Here's how the part is built. I have some questions about the finished solid (model axes, mm). Round coordinates to 2 decimals unless told otherwise and drop trailing zeros. Order: outer loops, then holes, each group sorted by start corner. A loop starts at its lowest first (then second) coordinate and runs counter-clockwise, first axis right, second up. Notation, with made-up numbers: (59, 68) - (69, 68) arc R4 ccw to (69, 75) - close; hole circle Ø6 at (82, 14). An arc over 180 degrees is marked (long way). Answer as a JSON object with one key per item and string values.
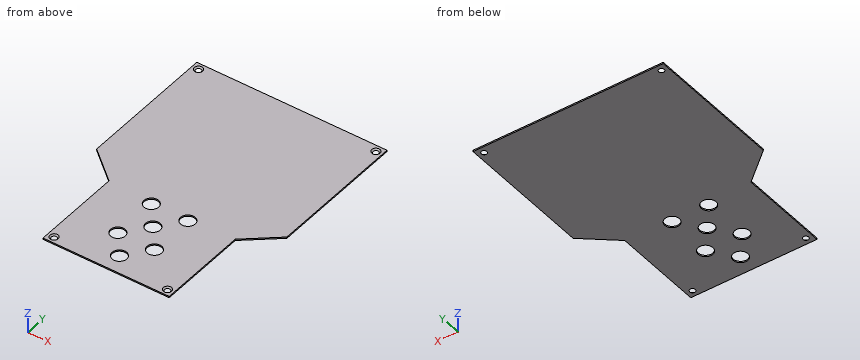
```python
from build123d import *

# Parameters (mm, degrees)
RESSALTO_EXTRUS_O1_DEPTH                     = 1.5
ESBO_O2_R                                    = 8
CORTE_EXTRUS_O1_DEPTH                        = 2.5
ESCAREADO_PARA_PARAFUSO_ALLEN_SEXTAV_2_COUNT = 2
ESCAREADO_PARA_PARAFUSO_ALLEN_SEXTAV_2_PITCH = 194
ESCAREADO_PARA_PARAFUSO_ALLEN_SEXTAV_3_COUNT = 2
ESCAREADO_PARA_PARAFUSO_ALLEN_SEXTAV_3_PITCH = 308.183386963
ESCAREADO_PARA_PARAFUSO_ALLEN_SEXTAV_4_COUNT = 2
ESCAREADO_PARA_PARAFUSO_ALLEN_SEXTAV_4_PITCH = 266.309969772


with BuildPart() as part:
    # Esboço1 → Ressalto-extrusão1 (new body)
    with BuildSketch(Plane.XY):
        Polygon((100.860947645, 140.996609125), (-107.139052355, 140.996609125), (-107.139052355, -8.842442963), (-72.139052355, -38.210930054), (-72.139052355, -137.003390875), (65.860947645, -137.003390875), (65.860947645, -38.210930054), (100.860947645, -8.842442963), align=None)
    extrude(amount=RESSALTO_EXTRUS_O1_DEPTH)

    # Esboço2 → Corte-extrusão1 (cut, through all)
    with BuildSketch(Plane.XY.offset(1.5)):
        with Locations((-3.139052355, -117.003390875)):
            Circle(ESBO_O2_R)
        with Locations((16.860947645, -42.003390875)):
            Circle(ESBO_O2_R)
        with Locations((-23.139052355, -92.003390875)):
            Circle(ESBO_O2_R)
        with Locations((-3.139052355, -67.003390875)):
            Circle(ESBO_O2_R)
        with Locations((16.860947645, -92.003390875)):
            Circle(ESBO_O2_R)
        with Locations((-23.139052355, -42.003390875)):
            Circle(ESBO_O2_R)
    extrude(amount=-CORTE_EXTRUS_O1_DEPTH, mode=Mode.SUBTRACT)

    # Esboço4 → Escareado para parafuso Allen sextavado escareado de M41 (revolve, cut)
    with BuildSketch(Plane(origin=(-100.139052355, 133.996609125, 1.5), x_dir=(0, -1, 0), z_dir=(1, 0, 0))):
        Polygon((0, 0), (0, 1.5), (2.25, 1.5), (2.25, 2.23), (4.48, 0), align=None)
    escareado_para_parafuso_allen_sextavado = revolve(axis=Axis((-100.139052355, 133.996609125, 7.85), (0, 0, -1)), mode=Mode.SUBTRACT)

    # Escareado para parafuso Allen sextav 2: Escareado para parafuso Allen sextavado escareado de M41 ×2
    with Locations(*[(i * ESCAREADO_PARA_PARAFUSO_ALLEN_SEXTAV_2_PITCH, 0, 0) for i in range(1, ESCAREADO_PARA_PARAFUSO_ALLEN_SEXTAV_2_COUNT)]):
        add(escareado_para_parafuso_allen_sextavado, mode=Mode.SUBTRACT)

    # Escareado para parafuso Allen sextav 3: Escareado para parafuso Allen sextavado escareado de M41 ×2
    with Locations(*[Vector(0.515926577, -0.856632808, 0) * (i * ESCAREADO_PARA_PARAFUSO_ALLEN_SEXTAV_3_PITCH) for i in range(1, ESCAREADO_PARA_PARAFUSO_ALLEN_SEXTAV_3_COUNT)]):
        add(escareado_para_parafuso_allen_sextavado, mode=Mode.SUBTRACT)

    # Escareado para parafuso Allen sextav 4: Escareado para parafuso Allen sextavado escareado de M41 ×2
    with Locations(*[Vector(0.131425797, -0.991326011, 0) * (i * ESCAREADO_PARA_PARAFUSO_ALLEN_SEXTAV_4_PITCH) for i in range(1, ESCAREADO_PARA_PARAFUSO_ALLEN_SEXTAV_4_COUNT)]):
        add(escareado_para_parafuso_allen_sextavado, mode=Mode.SUBTRACT)


solid = part.part
```
1. Imagine slicing it at D-D (x = 76). List the corners of the cut face in (y, z) for me, plus the area to 3 significant figures.
Responses:
{"outline": "(-29.7, 0) - (141, 0) - (141, 1.5) - (-29.7, 1.5) - close", "area": "256 mm2"}
2. For P1, Ø14.5, axis at x = -23.14, y = -42, coming from the -Z side, with a flat end and sliding along its axis, tell me the tip position at first contact or that it passes through.
Responses:
{"P1": "through"}
3. Imagine slicing it at B-B (z = 1.2). Give the number of separate pieces and of enclosed holes in the cut face, plus the area to 3 significant figures.
Responses:
{"separate pieces": "1", "enclosed holes": "10", "area": "48,500 mm2"}
4. Imagine slicing it at C-C (x = -87). List the corners of the cut face in (y, z) for me, plus the area to 3 significant figures.
Responses:
{"outline": "(-25.74, 0) - (141, 0) - (141, 1.5) - (-25.74, 1.5) - close", "area": "250 mm2"}
5. Imagine slicing it at A-A (x = -4). List the corners of the cut face in (y, z) for me.
Responses:
{"outline": "(-137, 0) - (-124.96, 0) - (-124.96, 1.5) - (-137, 1.5) - close; (-109.05, 0) - (-74.96, 0) - (-74.96, 1.5) - (-109.05, 1.5) - close; (-59.05, 0) - (141, 0) - (141, 1.5) - (-59.05, 1.5) - close"}
6. If I drill on L1, parallel to Y at x = 20, z = 0.25; L2, parallel to Y at x = 3, z = 0.25; L3, parallel to Y at x = 60, z = 0.8, over which ranges is the centre line in solid material (lowest first)? Write a range as [from, to].
Responses:
{"L1": "[-137, -99.36], [-84.64, -49.36], [-34.64, 141]", "L2": "[-137, -122.13], [-111.87, -72.13], [-61.87, 141]", "L3": "[-137, -133.61], [-126.4, 141]"}
